```python
from build123d import *

# Parameters (mm, degrees)
SKETCH2_W           = 12
SKETCH2_H           = 22
BOSS_EXTRUDE1_DEPTH = 22
SKETCH3_R           = 6
SKETCH3_R_2         = 2.45
BOSS_EXTRUDE2_DEPTH = 4
SKETCH4_W           = 12
SKETCH4_H           = 2
BOSS_EXTRUDE3_DEPTH = 5
SKETCH5_W           = 12
SKETCH5_H           = 2
BOSS_EXTRUDE4_DEPTH = 5
FILLET1_R           = 1
FILLET2_R           = 0.5


with BuildPart() as part:
    # Sketch2 → Boss-Extrude1 (new body)
    with BuildSketch(Plane(origin=(0, 0, 0), x_dir=(1, 0, 0), z_dir=(0, 1, 0))):
        with Locations((6, -42.720930233)):
            Rectangle(SKETCH2_W, SKETCH2_H)
    extrude(amount=BOSS_EXTRUDE1_DEPTH)

    # Sketch3 → Boss-Extrude2 (add)
    with BuildSketch(Plane(origin=(0, 22, 0), x_dir=(1, 0, 0), z_dir=(0, 1, 0))):
        with Locations(Location((6, -47.720930233, 0), (0, 0, 270))):
            Circle(SKETCH3_R)
        with Locations(Location((6, -47.720930233, 0), (0, 0, 270))):
            Circle(SKETCH3_R_2, mode=Mode.SUBTRACT)
    extrude(amount=BOSS_EXTRUDE2_DEPTH)

    # Sketch4 → Boss-Extrude3 (add)
    with BuildSketch(Plane.XY.offset(53.720930233)):
        with Locations((6, 17)):
            Rectangle(SKETCH4_W, SKETCH4_H)
    extrude(amount=BOSS_EXTRUDE3_DEPTH)

    # Sketch5 → Boss-Extrude4 (add)
    with BuildSketch(Plane(origin=(0, 0, 31.720930233), x_dir=(-1, 0, 0), z_dir=(0, 0, -1))):
        with Locations((-6, 17)):
            Rectangle(SKETCH5_W, SKETCH5_H)
    extrude(amount=BOSS_EXTRUDE4_DEPTH)

    # Fillet1
    fillet1_edges = [part.edges().sort_by_distance(p)[0] for p in [
        (0, 17, 58.720930233),
        (12, 17, 58.720930233),
        (12, 17, 26.720930233),
        (0, 17, 26.720930233),
    ]]
    fillet(fillet1_edges, radius=FILLET1_R)

    # Fillet2
    fillet2_edges = [part.edges().sort_by_distance(p)[0] for p in [
        (12, 8, 53.720930233),
        (0, 8, 53.720930233),
        (0, 8, 31.720930233),
        (12, 8, 31.720930233),
        (0, 20, 31.720930233),
        (12, 20, 31.720930233),
        (12, 20, 53.720930233),
        (0, 20, 53.720930233),
    ]]
    fillet(fillet2_edges, radius=FILLET2_R)


solid = part.part
```
Could you check a few things on this model? Use its own coordinates, in mm. A direction names the side the tool comes from. Round coordinates to 2 decimals unless told otherwise and drop trailing zeros. Loops run counter-clockwise (first coordinate to the right, second up) from the corner with the lowest first, then second, coordinate; pieces in that order, holes last. Notation, with made-up numbers: M 1,-27 L 40,-27 A5 cw 40,-22 Z; hole C 76,35 d6. An arc over 180 degrees is marked long. Answer as CSV lines item,"result".
1) Imagine slicing it at C-C on z = 30.5. List the corners of the cut face in (x, y) for me, and give its area (3 significant figures).
From the geometry:
outline,"M 0,16 L 12,16 L 12,18 L 0,18 Z"
area,"24.0 mm^2"
2) Imagine slicing it at B-B on y = 3.5. List the corners of the cut face in (x, z) for me, and give its area (3 significant figures).
From the geometry:
outline,"M 0,32.22 A0.5 ccw 0.5,31.72 L 11.5,31.72 A0.5 ccw 12,32.22 L 12,53.22 A0.5 ccw 11.5,53.72 L 0.5,53.72 A0.5 ccw 0,53.22 Z"
area,"264 mm^2"
3) For pin 1 Ø3.5 at (x, y) = (6, 10.5) entering from -Z; pin 2 Ø5.5 at (x, y) = (4, 8.5) entering from +Z; pin 3 Ø4.5 at (x, z) = (6.5, 30.5) entering from +Y, each with a flat end and sliding along its axis, tell me the tip position at first contact or that it passes through.
From the geometry:
pin 1,"z = 31.72"
pin 2,"z = 53.72"
pin 3,"y = 22"
4) Imagine slicing it at D-D on x = 10. List the corners of the cut face in (y, z) for me, and give its area (3 significant figures).
From the geometry:
outline,"M 0,31.72 L 16,31.72 L 16,26.72 L 18,26.72 L 18,31.72 L 22,31.72 L 22,43.25 L 26,43.25 L 26,52.19 L 22,52.19 L 22,53.72 L 18,53.72 L 18,58.72 L 16,58.72 L 16,53.72 L 0,53.72 Z"
area,"540 mm^2"
5) If I drill on probe 1 along Z at (x, y) = (0.5, 7.5); probe 2 along Y at (x, z) = (11.5, 33.5); probe 3 along Z at (x, y) = (4, 22.5), over which ranges is the centre line in solid material (lowest first)?
From the geometry:
probe 1,"31.72 to 53.72"
probe 2,"0 to 22"
probe 3,"42.06 to 46.31, 49.14 to 53.38"
6) Imagine slicing it at A-A on x = 4. List the corners of the cut face in (y, z) for me.
From the geometry:
outline,"M 0,31.72 L 16,31.72 L 16,26.72 L 18,26.72 L 18,31.72 L 22,31.72 L 22,42.06 L 26,42.06 L 26,46.31 L 22,46.31 L 22,49.14 L 26,49.14 L 26,53.38 L 22,53.38 L 22,53.72 L 18,53.72 L 18,58.72 L 16,58.72 L 16,53.72 L 0,53.72 Z"
7) Which directions (+Z, -Z, +X, -X, +Y, -Y) give clear straight access to the entire face, cutting with the end or side of a thin tool? Please do faces 1 (the flat face through (6, 8, 31.721)), 2 (the cylindrical face through (7.802, 23.972, 53.444)), 3 (the flat face through (11, 22, 52)).
From the geometry:
face 1,"-Z, +X, -X, -Y"
face 2,"+Y"
face 3,"+Z, +X, +Y"
